Work out the finished part from the listing and answer in its coordinate system (mm). A direction names the side the tool comes from. Give positions to 0.01 mm unless a question says otherwise; leave off trailing zeros. Write each loop counter-clockwise with the first axis right and the second up, starting at its lowest first coordinate (ties: lowest second). Pieces come first, ordered by that corner, then holes.
1) Determine the mould class of faces 4 (the face through (9, -1, -71.425)), 5 (the face through (56.31, -0.36, -23.24)), 6 (the face through (12.09, -0.36, -13.53)) for opening direction X: pulls with the +X half, pulls with the -X half, needs draft (parallel to the pull), parting line crosses it, or undercut.
2) Straight lines are drawn through the part: probe 1 along Z at (x, y) = (30.5, -51); probe 2 along Y at (x, z) = (-16, -35.5); probe 3 along X at (y, z) = (-20, -56.5). For each, find the intervals that lie inside material, in ascending order.
3) Find section B-B (y = 0). Determine the outline of the cut face in (x, z) (3 decimals), plus the area to 3 significant figures.
4) Find section D-D (x = 11). Determine the outline of the cut face in (y, z), plus the area to 3 significant figures.
5) Find section A-A (z = -60). Determine the outline of the cut face in (x, y).
6) A tool of negligible diameter and unlimited length cuts with its end or side. For faces 1 (the face through (11, 44, -52.375)), 2 (the face through (70, 0, 0)), 3 (the face through (70, 0, -19.025)), from which of +Z, -Z, +X, -X, +Y, -Y can it reach the whole face along a straight path? Write none if from no direction.
7) Given pin 1 Ø8 at (x, z) = (6, -22) entering from +Y; pin 2 Ø6 at (x, y) = (60, 0.5) entering from +Z; pin 3 Ø8 at (y, z) = (-13, -46.5) entering from -X, each flat-ended and moving along its own axis, determine where each tip first touches the part or whether it passes through.
8) Find section C-C (x = 78). Determine the outline of the cut face in (y, z), plus the area to 3 significant figures.
```python
from build123d import *

# Parameters (mm, degrees)
F1_DEPTH = 63.5
F0_W     = 19.05
F0_H     = 19.05
F0_W_2   = 3.2533031947
F0_H_2   = 19.0246
F0_W_3   = 25.4
F2_DEPTH = 25.4
F4_R     = 5.08


with BuildPart() as f1:
    # F0 (on Front) → F1 (new body, symmetric)
    with BuildSketch(Plane.XZ):
        Polygon((32.2343749046, -52.3748), (-31.2656250954, -52.3748), (-31.2656250954, -71.4248), (51.2843749046, -71.4248), (51.2843749046, -52.3748), align=None)
    extrude(amount=F1_DEPTH, both=True)

    # F0 (on Front) → F2 (join, symmetric)
    with BuildSketch(Plane.XZ):
        with BuildLine():
            ThreePointArc((67.08107171, 0), (11.3693304709, -13.9099433247), (-31.2656250954, -52.3748))
            Line((-31.2656250954, -52.3748), (32.2343749046, -52.3748))
            Line((32.2343749046, -52.3748), (32.2343749046, -33.3248))
            ThreePointArc((32.2343749046, -33.3248), (42.9728025203, -9.6721882708), (67.08107171, 0))
        make_face()
        with BuildLine():
            Line((67.08107171, -19.0246), (67.08107171, 0))
            ThreePointArc((67.08107171, 0), (42.9728025203, -9.6721882708), (32.2343749046, -33.3248))
            Line((32.2343749046, -33.3248), (51.2843749046, -33.3248))
            ThreePointArc((51.2843749046, -33.3248), (56.4270660079, -23.1306668495), (67.08107171, -19.0246))
        make_face()
        with Locations((41.7593749046, -42.8498)):
            Rectangle(F0_W, F0_H)
        with Locations((68.7077233073, -9.5123)):
            Rectangle(F0_W_2, F0_H_2)
        with Locations((83.0343749046, -9.5123)):
            Rectangle(F0_W_3, F0_H_2)
    extrude(amount=F2_DEPTH, both=True)

    # F0 (on Front) → F3 (revolve)
    with BuildSketch(Plane.XZ):
        Polygon((95.7343749046, 4.7752), (95.7343749046, 0), (95.7343749046, -19.0246), (95.7343749046, -23.7998), (121.1343749046, -23.7998), (121.1343749046, 4.7752), align=None)
    revolve(axis=Axis((95.7343749046, 0, -9.5123), (0, 0, -1)))

    # F4
    f4_edges = [f1.edges().sort_by_distance(p)[0] for p in [
        (-31.265625, -63.5, -61.8998),
        (51.284375, -63.5, -61.8998),
        (51.284375, 63.5, -61.8998),
        (-31.265625, 63.5, -61.8998),
    ]]
    fillet(f4_edges, radius=F4_R)


solid = f1.part
```
Results:
1. face 4: needs draft
1. face 5: undercut
1. face 6: pulls with the -X half
2. probe 1: z = -71.42 to -52.37
2. probe 2: y = -25.4 to 25.4
2. probe 3: x = -31.27 to 51.28
3. outline: (-31.266, -71.425) - (51.284, -71.425) - (51.284, -33.325) arc R15.875 cw to (67.081, -19.025) - (70.334, -19.025) - (70.334, -23.8) - (121.134, -23.8) - (121.134, 4.775) - (70.334, 4.775) - (70.334, 0) - (67.081, 0) arc R118.523 ccw to (-31.266, -52.375) - close
3. area: 6,230 mm2
4. outline: (-63.5, -71.42) - (63.5, -71.42) - (63.5, -52.37) - (25.4, -52.37) - (25.4, -14.11) - (-25.4, -14.11) - (-25.4, -52.37) - (-63.5, -52.37) - close
4. area: 4,360 mm2
5. outline: (-31.27, -58.42) arc R5.08 ccw to (-26.19, -63.5) - (46.2, -63.5) arc R5.08 ccw to (51.28, -58.42) - (51.28, 58.42) arc R5.08 ccw to (46.2, 63.5) - (-26.19, 63.5) arc R5.08 ccw to (-31.27, 58.42) - close
6. face 1: +Z, +X, -X, +Y
6. face 2: +Z, -X
6. face 3: -Z
7. pin 1: stops at y = 25.4
7. pin 2: stops at z = -0.07
7. pin 3: stops at x = -29.98
8. outline: (-25.4, -19.02) - (-18.18, -19.02) - (-18.18, -23.8) - (18.18, -23.8) - (18.18, -19.02) - (25.4, -19.02) - (25.4, 0) - (18.18, 0) - (18.18, 4.78) - (-18.18, 4.78) - (-18.18, 0) - (-25.4, 0) - close
8. area: 1,310 mm2
